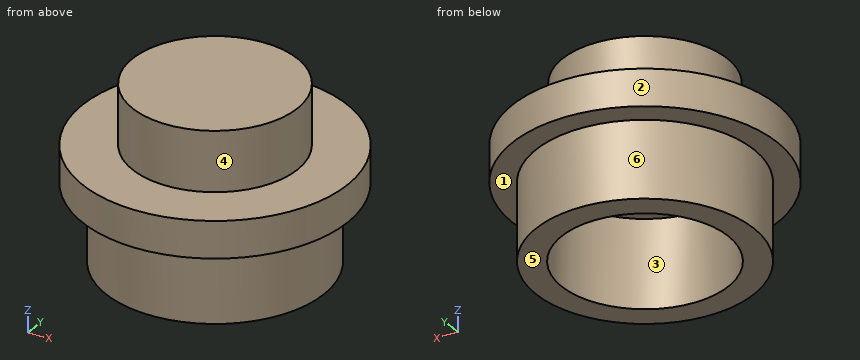
```python
from build123d import *

# Parameters (mm, degrees)
F0_R     = 3.2385
F1_DEPTH = 2.286
F2_R     = 3.937
F3_DEPTH = 1.0922
F4_R     = 2.4511
F5_DEPTH = 1.778
F6_T     = -0.762


with BuildPart() as f1:
    # F0 (on Top) → F1 (new body)
    with BuildSketch(Plane.XY):
        Circle(F0_R)
    extrude(amount=F1_DEPTH)

    # F2 (on face) → F3 (join)
    with BuildSketch(Plane.XY.offset(2.286)):
        Circle(F2_R)
    extrude(amount=F3_DEPTH)

    # F4 (on face) → F5 (join)
    with BuildSketch(Plane.XY.offset(3.3782)):
        Circle(F4_R)
    extrude(amount=F5_DEPTH)

    # F6
    f6_openings = [f1.faces().sort_by_distance(p)[0] for p in [
        (0, 0, 0),
    ]]
    offset(amount=F6_T, openings=f6_openings, kind=Kind.INTERSECTION)


solid = f1.part
```
For this review, take the finished solid that the model builds, in its own axes (mm). Face numbers are marked on the shaded views. A direction names the side the tool comes from. Round coordinates to 2 decimals unless told otherwise and drop trailing zeros. Order: outer loops, then holes, each group sorted by start corner. A loop starts at its lowest first (then second) coordinate and runs counter-clockwise, first axis right, second up.
Q1. Mouldability with a two-part tool opening along Y and no side actions: class the marked faces 1, 2 and 3 as pulls with the +Y half, pulls with the -Y half, needs draft (parallel to the pull), parting line crosses it, or undercut.
Findings below:
face 1: needs draft
face 2: parting line crosses it
face 3: undercut
Q2. Machinability: for the marked faces 4, 5 and 6, which of the approach directions +Z, -Z, +X, -X, +Y, -Y give a long, thin tool a straight path to every point of the face, cutting with its end or side? Answer none if there is none.
Findings below:
face 4: +Z
face 5: -Z, +X, -X, +Y, -Y
face 6: -Z
Q3. We need section D-D, the plane x = -2.25. Give the boundary of the cut face in (y, z).
Findings below:
outline: (-3.23, 2.29) - (-2.33, 2.29) - (-2.33, 0) - (-1.03, 0) - (-1.03, 2.62) - (1.03, 2.62) - (1.03, 0) - (2.33, 0) - (2.33, 2.29) - (3.23, 2.29) - (3.23, 3.38) - (0.97, 3.38) - (0.97, 5.16) - (-0.97, 5.16) - (-0.97, 3.38) - (-3.23, 3.38) - close
Q4. Wall thickness on line 1 (Y direction, x = 0, z = 1.3); line 2 (Y direction, x = 0, z = 2.95); line 3 (X direction, y = 1, z = 2.55): over which ranges is each line inside the solid? List them lowest first.
Findings below:
line 1: y = -3.24 to -2.48, 2.48 to 3.24
line 2: y = -3.94 to -1.69, 1.69 to 3.94
line 3: x = -3.81 to -2.27, 2.27 to 3.81
Q5. We need section C-C, the plane z = 1. Give the boundary of the cut face in (x, y).
Findings below:
outline: circle Ø6.48 at (0, 0); hole circle Ø4.95 at (0, 0)
Q6. Insertion check: P1, Ø2, axis at x = -2.5, z = 3.5, coming from the -Y side; P2, Ø1.5, axis at x = 0, y = -1, coming from the -Z side; P3, Ø1, axis at x = -1.5, z = 4, coming from the -Y side. Each pin has a flat end and moves straight along its axis. Give the tip position at first contact, or say it passes through.
Findings below:
P1: stops at y = -3.64
P2: stops at z = 2.62
P3: stops at y = -2.24
Q7. We need section A-A, the plane x = 0. Give the boundary of the cut face in (y, z).
Findings below:
outline: (-3.94, 2.29) - (-3.24, 2.29) - (-3.24, 0) - (-2.48, 0) - (-2.48, 2.62) - (-1.69, 2.62) - (-1.69, 4.39) - (1.69, 4.39) - (1.69, 2.62) - (2.48, 2.62) - (2.48, 0) - (3.24, 0) - (3.24, 2.29) - (3.94, 2.29) - (3.94, 3.38) - (2.45, 3.38) - (2.45, 5.16) - (-2.45, 5.16) - (-2.45, 3.38) - (-3.94, 3.38) - close
